Autodesk Inventor part; units mm, degrees
ref_plane "nt_XY" through (0, 0, 0) normal (1, 0, 0) x (0, 0, -1)
ref_plane "nt_YZ" through (0, 0, 0) normal (0, 0, -1) x (0, 1, 0)
ref_plane "nt_ZX" through (0, 0, 0) normal (0, 1, 0) x (1, 0, 0)
sketch "B" plane through (0, 0, 0) normal (1, 0, 0) x (0, 1, 0)
  line L0 (-2.0207, 3.5) -> (-4.0415, 0)
  line L1 (-4.0415, 0) -> (-2.0207, -3.5)
  line L2 (-2.0207, -3.5) -> (2.0207, -3.5)
  line L3 (2.0207, -3.5) -> (4.0415, 0)
  line L4 (4.0415, 0) -> (2.0207, 3.5)
  line L5 (2.0207, 3.5) -> (-2.0207, 3.5)
extrude "Extrusion1" add sketch "B" along normal mid plane 3.2
sketch "Sketch_2" plane through (0, 0, 0) normal (0, 0, 1) x (1, 0, 0)
  line L0 (1.6, 0) -> (-1.6, 0)
  line L1 (-1.6, 0) -> (-1.6, 2)
  line L2 (-1.6, 2) -> (-1.221, 1.621)
  line L3 (-1.221, 1.621) -> (1.221, 1.621)
  line L4 (1.221, 1.621) -> (1.6, 2)
  line L5 (1.6, 2) -> (1.6, 0)
  line L6 (1.6, 0) -> (-1.6, 0)
revolve "Revolution1" cut sketch "Sketch_2" angle 360 about axis through (1.6, 0, 0) along (1, 0, 0)
thread "Thread1"
sketch "Sketch_3" plane through (0, 0, 0) normal (0, 0, 1) x (1, 0, 0)
  line L0 (50, 0) -> (-50, 0)
  line L1 (-6.6, 6.94) -> (-6.6, 1)
  line L2 (-6.6, 1) -> (-1.6, 1)
  line L3 (-1.6, 1) -> (-1.6, 2.94)
  line L4 (-1.6, 2.94) -> (0, 5.7113)
  line L5 (0, 5.7113) -> (1.6, 2.94)
  line L6 (1.6, 2.94) -> (1.6, 1)
  line L7 (1.6, 1) -> (6.6, 1)
  line L8 (6.6, 1) -> (6.6, 6.94)
  line L9 (6.6, 6.94) -> (-6.6, 6.94)
revolve "Revolution2" cut sketch "Sketch_3" angle 360 about axis through (50, 0, 0) along (1, 0, 0)
ref_plane "nt_XY" through (0, 0, 0) normal (1, 0, 0) x (0, 0, -1)
ref_plane "nt_YZ" through (0, 0, 0) normal (0, 0, -1) x (0, 1, 0)
ref_plane "nt_ZX" through (0, 0, 0) normal (0, 1, 0) x (1, 0, 0)
ref_plane "ntj_XY" through (1.6, 0, 0) normal (1, 0, 0) x (0, 0, -1)
ref_plane "ntj_YZ" through (1.6, 0, 0) normal (0, 0, -1) x (0, 1, 0)
ref_plane "ntj_ZX" through (1.6, 0, 0) normal (0, 1, 0) x (1, 0, 0)
properties part number "NTJ-010A_CJ2"
CAD build for the part. Positions are in the model's coordinates, mm. Coordinates: 2 decimals unless noted, no trailing zeros. Write each loop counter-clockwise with the first axis right and the second up, starting at its lowest first coordinate (ties: lowest second). Pieces come first, ordered by that corner, then holes. Notation, with made-up numbers: M -7,-15.75 L 3,-15.75 A26 cw 3,14.25 Z; hole C 42,33 d10. An arc over 180 degrees is marked long. Return JSON: item names as keys, results as strings.
Item 1: Slice it at A-A, the plane x = -0.75. Write the cut outline in (y, z).
Findings below:
{"outline": "M -4.04,0 L -2.02,-3.5 L 2.02,-3.5 L 4.04,0 L 2.02,3.5 L -2.02,3.5 Z; hole C 0,0 d3.24"}
Item 2: Two-plate mould, pull along Z, no slides. Class faces 1 (the flat face through (0, -3, 1.8)), 2 (the cylindrical face through (0.017, 0.748, -1.438)), 3 (the flat face through (-1.6, 2, -1)), 4 (the flat face through (0, 3, -1.8)): +Z half, -Z half, draft (parallel to the pull), parting line (faces both ways), or undercut.
Findings below:
{"face 1": "+Z half", "face 2": "undercut", "face 3": "draft", "face 4": "-Z half"}
Item 3: Drop a flat-ended pin along its axis: pin 1 Ø1.9 at (y, z) = (0, 0) entering from +X. Give the stop position or say it passes through.
Findings below:
{"pin 1": "passes through"}
Item 4: Slice it at B-B, the plane y = 0. Write the cut outline in (x, z).
Findings below:
{"outline": "M -1.6,-2.94 L -1.28,-3.5 L 1.28,-3.5 L 1.6,-2.94 L 1.6,-2 L 1.22,-1.62 L -1.22,-1.62 L -1.6,-2 Z; M -1.6,2 L -1.22,1.62 L 1.22,1.62 L 1.6,2 L 1.6,2.94 L 1.28,3.5 L -1.28,3.5 L -1.6,2.94 Z"}
Item 5: Probe line 1 (Z direction, x = 0.45, y = 0.25); line 2 (Y direction, x = 0.35, z = -1); line 3 (Y direction, x = -0.3, z = 1.25). List the from-to ranges inside material, lowest first. Write a range as from..to.
Findings below:
{"line 1": "z = -3.5..-1.6, 1.6..3.5", "line 2": "y = -3.46..-1.28, 1.28..3.46", "line 3": "y = -3.32..-1.03, 1.03..3.32"}
